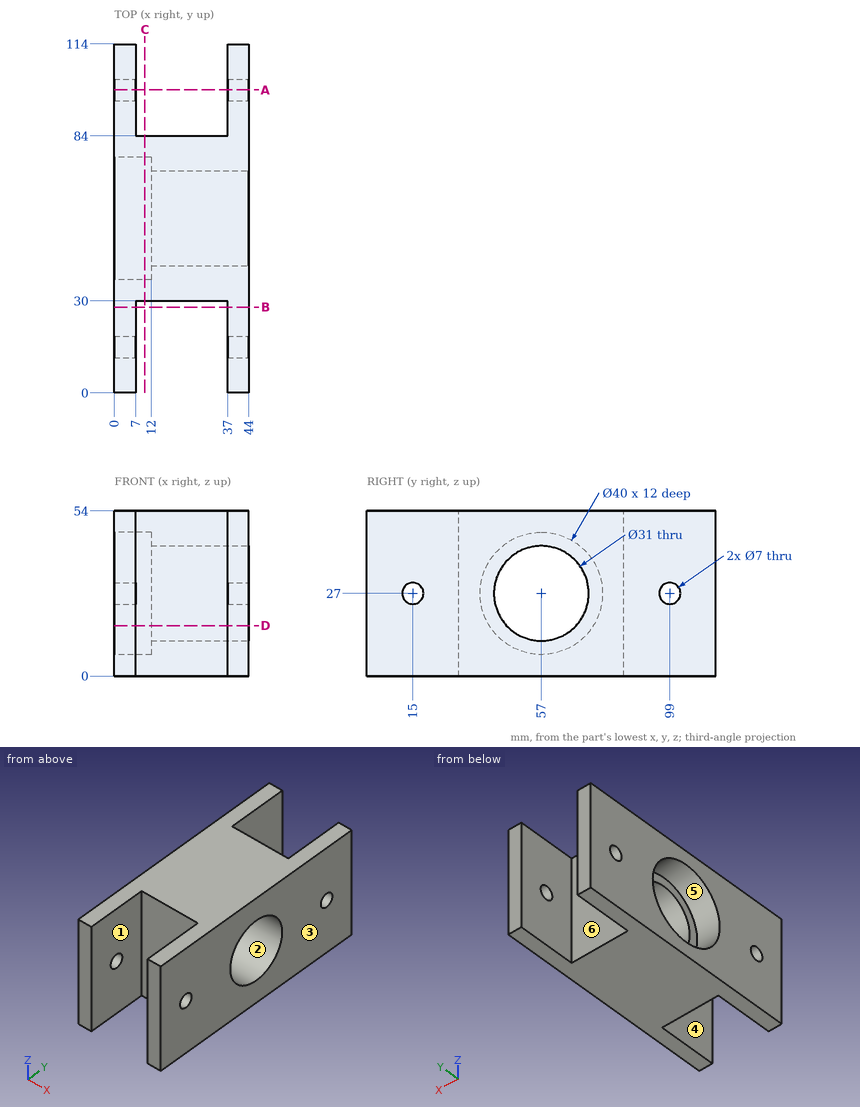
Verification items for this drawing (mm, ordinates from the low corner). A direction names the side the tool comes from. Give positions to 0.01 mm unless a question says otherwise; leave off trailing zeros. Write each loop counter-clockwise with the first axis right and the second up, starting at its lowest first coordinate (ties: lowest second). Pieces come first, ordered by that corner, then holes. Notation, with made-up numbers: M -37,29 L 14,29 A21 ccw 14,35 Z; hole C 46.25,-15.5 d9. An arc over 180 degrees is marked long. Use one line per item in the form item = value.
(1) Draft check along X on the marked faces 1, 2 and 3. Enter one of: pulls with the +X half, pulls with the -X half, needs draft (parallel to the pull), parting line crosses it, or undercut.
Answer block:
face_1 = undercut
face_2 = needs draft
face_3 = pulls with the +X half
(2) Tool access check on the marked faces 4, 5 and 6. Record the directions out of +Z, -Z, +X, -X, +Y, -Y that give a thin tool (end or side, any length) a straight path to the whole face; none if there is none.
Answer block:
face_4 = +Z, -Z, -Y
face_5 = -X
face_6 = +Z, -Z, +Y
(3) Section check B-B on y = 28. Record the boundary of the cut face in (x, z).
Answer block:
outline = M 0,0 L 7,0 L 7,54 L 0,54 Z; M 37,0 L 44,0 L 44,54 L 37,54 Z
(4) Section check D-D on z = 16.5. Record the boundary of the cut face in (x, y), plus the area to 3 significant figures.
Answer block:
outline = M 0,0 L 7,0 L 7,30 L 37,30 L 37,0 L 44,0 L 44,45.6 L 12,45.6 L 12,39.98 L 0,39.98 Z; M 0,74.02 L 12,74.02 L 12,68.4 L 44,68.4 L 44,114 L 37,114 L 37,84 L 7,84 L 7,114 L 0,114 Z
area = 2,080 mm2
(5) Depth check by flat-ended pin: P1, Ø2, axis at x = 30, z = 26, coming from the -Y side; P2, Ø24, axis at x = 23, z = 34, coming from the +Y side. Enter the tip coordinate at first touch or a pass-through.
Answer block:
P1 = 30
P2 = 84
(6) Section check A-A on y = 99. Record the boundary of the cut face in (x, z).
Answer block:
outline = M 0,0 L 7,0 L 7,23.5 L 0,23.5 Z; M 0,30.5 L 7,30.5 L 7,54 L 0,54 Z; M 37,0 L 44,0 L 44,23.5 L 37,23.5 Z; M 37,30.5 L 44,30.5 L 44,54 L 37,54 Z
(7) Material ranges on line 1 along Y through (x, z) = (3, 27); line 2 along Y through (x, z) = (38.75, 27); line 3 along X through (y, z) = (19, 26.5), recorded low to high.
Answer block:
line_1 = 0 to 11.5, 18.5 to 37, 77 to 95.5, 102.5 to 114
line_2 = 0 to 11.5, 18.5 to 41.5, 72.5 to 95.5, 102.5 to 114
line_3 = 0 to 7, 37 to 44
(8) Section check C-C on x = 10. Record the boundary of the cut face in (y, z), plus the area to 3 significant figures.
Answer block:
outline = M 30,0 L 84,0 L 84,54 L 30,54 Z; hole C 57,27 d40
area = 1,660 mm2
